Check sheet for the modelled part. Datum: model origin and axes. Units: mm. Face numbers are marked on the shaded views. A direction names the side the tool comes from. Round coordinates to 2 decimals unless told otherwise and drop trailing zeros. Order: outer loops, then holes, each group sorted by start corner. A loop starts at its lowest first (then second) coordinate and runs counter-clockwise, first axis right, second up. Notation, with made-up numbers: (-27.5, -39) -> (-1.5, -39) arc R17 cw to (-1.5, -33) -> close; hole circle Ø1 at (47.5, 43.25). An arc over 180 degrees is marked (long way). Answer in a Markdown table with one row per item.
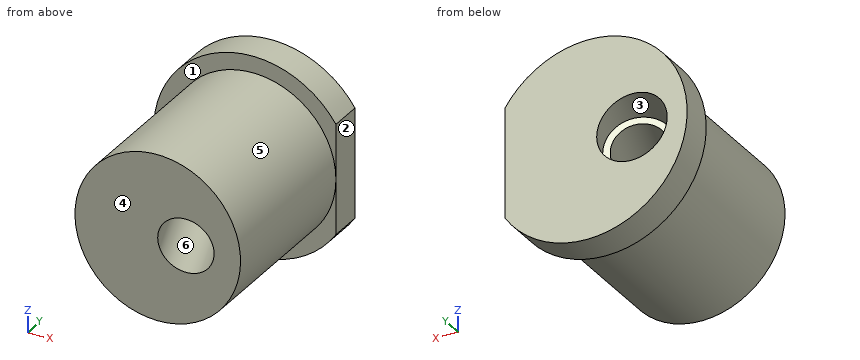
from build123d import *

# Parameters (mm, degrees)
SKETCH4_W          = 19.505959246
SKETCH4_H          = 52.283096245
CUT_EXTRUDE1_DEPTH = 18


with BuildPart() as part:
    # Sketch1 → Revolve1 (revolve)
    with BuildSketch(Plane.XY, mode=Mode.PRIVATE) as revolve1_sk:
        Polygon((0, 0), (0, 60), (30, 60), (30, 50), (25, 50), (25, 0), align=None)
    revolve(revolve1_sk.sketch.rotate(Axis((0, 0, 0), (0, 1, 0)), 90), axis=Axis((0, 0, 0), (0, 1, 0)))

    # Sketch4 → Cut-Extrude1 (cut)
    with BuildSketch(Plane(origin=(0, 60, 0), x_dir=(1, 0, 0), z_dir=(0, 1, 0))):
        with Locations((34.752979623, -0.356273229)):
            Rectangle(SKETCH4_W, SKETCH4_H)
    extrude(amount=-CUT_EXTRUDE1_DEPTH, mode=Mode.SUBTRACT)

    # Sketch5 → Cut-Revolve1 (revolve, cut)
    with BuildSketch(Plane.XY, mode=Mode.PRIVATE) as cut_revolve1_sk:
        Polygon((-23.756678995, 88.624497165), (16.900700587, -23.08073517), (24.418241553, -20.344574023), (-16.239138029, 91.360658312), align=None)
    revolve(cut_revolve1_sk.sketch.rotate(Axis((-23.756678995, 88.624497165, 0), (0.34202014332567277, -0.939692620785907, 0)), 180), axis=Axis((-23.756678995, 88.624497165, 0), (0.34202014332567277, -0.939692620785907, 0)), mode=Mode.SUBTRACT)

    # Sketch6 → Cut-Revolve2 (revolve, cut)
    with BuildSketch(Plane.XY):
        Polygon((-9.693720942, 50), (-17.792178214, 72.250328486), (-8.395252006, 75.670529919), (-0.296794735, 53.420201433), (0.387245552, 51.540816192), (-9.009680656, 48.120614758), align=None)
    revolve(axis=Axis((-9.693720942, 50, 0), (-0.3420201433256727, 0.939692620785907, 0)), mode=Mode.SUBTRACT)


solid = part.part
Item 1: Set-up check for the marked faces 1 and 2: record each of +Z, -Z, +X, -X, +Y, -Y from which the full face is reachable in a straight line by a thin tool's end or side.
Result sheet:
| item | result |
|---|---|
| face 1 | -Y |
| face 2 | +Z, -Z, +X, +Y, -Y |
Item 2: Depth check by flat-ended pin: P1, Ø4, axis at y = 40, z = -21.5, coming from the +X side; P2, Ø8, axis at x = 4, z = -7, coming from the -Y side; P3, Ø1.5, axis at x = 3.5, y = 14.5, coming from the +Z side; P4, Ø4, axis at x = 10, y = 37.5, coming from the -Z side. Enter the tip coordinate at first touch or a pass-through.
Result sheet:
| item | result |
|---|---|
| P1 | stops at x = 15.64 |
| P2 | stops at y = 0 |
| P3 | stops at z = 24.85 |
| P4 | stops at z = -23.69 |
Item 3: Scan lines: line 1 (Y direction, x = -26.5, z = -10); line 2 (X direction, y = 24.5, z = -6); line 3 (Z direction, x = 11.5, y = 10). Record each from-to range of solid material in increasing order. Write a range as [from, to].
Result sheet:
| item | result |
|---|---|
| line 1 | y = [50, 60] |
| line 2 | x = [-24.27, -6.05], [5.21, 24.27] |
| line 3 | z = [-22.2, -5.01], [5.01, 22.2] |
Item 4: Cross-section at A-A (z = -4.5). Record the boundary of the cut face in (x, y).
Result sheet:
| item | result |
|---|---|
| outline | (-29.66, 50) -> (-24.59, 50) -> (-24.59, 0) -> (1.46, 0) -> (-15.23, 45.86) -> (-17.4, 45.07) -> (-22.84, 60) -> (-29.66, 60) -> close; (-3.83, 60) -> (-0.62, 51.17) -> (-2.8, 50.38) -> (15.54, 0) -> (24.59, 0) -> (24.59, 50) -> (25, 50) -> (25, 60) -> close |
Item 5: Cross-section at B-B (x = 21). Record the boundary of the cut face in (y, z).
Result sheet:
| item | result |
|---|---|
| outline | (0, -13.56) -> (50, -13.56) -> (50, -21.42) -> (60, -21.42) -> (60, 21.42) -> (50, 21.42) -> (50, 13.56) -> (0, 13.56) -> close |
Item 6: Mould release check, pull along Y, two halves, no side actions. Record for the marked faces 3, 4, 5 and 6: pulls with the +Y half, pulls with the -Y half, needs draft (parallel to the pull), parting line crosses it, or undercut.
Result sheet:
| item | result |
|---|---|
| face 3 | undercut |
| face 4 | pulls with the -Y half |
| face 5 | needs draft |
| face 6 | undercut |
Item 7: Cross-section at C-C (z = -20). Record the boundary of the cut face in (x, y), and give its area (3 significant figures).
Result sheet:
| item | result |
|---|---|
| outline | (-22.36, 50) -> (-15, 50) -> (-15, 0) -> (15, 0) -> (15, 50) -> (22.36, 50) -> (22.36, 60) -> (-22.36, 60) -> close |
| area | 1,950 mm^2 |
